```python
from build123d import *

# Parameters (mm, degrees)
SKETCH1_W           = 279.4
SKETCH1_H           = 376.174
BOSS_EXTRUDE1_DEPTH = 2.54
SKETCH2_W           = 28.448
SKETCH2_H           = 19.05
CUT_EXTRUDE1_DEPTH  = 235.305913645


with BuildPart() as part:
    # Sketch1 → Boss-Extrude1 (new body)
    with BuildSketch(Plane(origin=(0, 0, 0), x_dir=(1, 0, 0), z_dir=(0, 1, 0))):
        Rectangle(SKETCH1_W, SKETCH1_H)
    extrude(amount=BOSS_EXTRUDE1_DEPTH)

    # Sketch2 → Cut-Extrude1 (cut, through all)
    with BuildSketch(Plane(origin=(0, 2.54, 0), x_dir=(1, 0, 0), z_dir=(0, 1, 0))):
        with Locations((-120.65, -105.537)):
            Rectangle(SKETCH2_W, SKETCH2_H)
        with Locations((-120.65, -162.687)):
            Rectangle(SKETCH2_W, SKETCH2_H)
        with Locations((-120.65, -48.387)):
            Rectangle(SKETCH2_W, SKETCH2_H)
        with Locations((-120.65, 8.763)):
            Rectangle(SKETCH2_W, SKETCH2_H)
        with Locations((-120.65, 65.913)):
            Rectangle(SKETCH2_W, SKETCH2_H)
        with Locations((120.65, 65.913)):
            Rectangle(SKETCH2_W, SKETCH2_H)
        with Locations((120.65, 8.763)):
            Rectangle(SKETCH2_W, SKETCH2_H)
        with Locations((120.65, -48.387)):
            Rectangle(SKETCH2_W, SKETCH2_H)
        with Locations((120.65, -105.537)):
            Rectangle(SKETCH2_W, SKETCH2_H)
        with Locations((120.65, -162.687)):
            Rectangle(SKETCH2_W, SKETCH2_H)
    extrude(amount=-CUT_EXTRUDE1_DEPTH, mode=Mode.SUBTRACT)


solid = part.part
```
Part model, mm, in its own coordinate system. Round coordinates to 2 decimals unless told otherwise and drop trailing zeros. Loops run counter-clockwise (first coordinate to the right, second up) from the corner with the lowest first, then second, coordinate; pieces in that order, holes last.
Item 1: Cut at A-A, the plane z = -61.5. Give the cut face in (x, y), then the cut area to 3 significant figures.
Item 2: Cut at B-B, the plane y = 0.8. State how many separate pieces and enclosed holes the cut face has, then the cut area to 3 significant figures.
Item 3: Drill centre lines: line 1 (Z direction, x = 116, y = 1.45); line 2 (X direction, y = 1.8, z = 155). Where is each one in solid material? Low to high.
A:
1. outline: (-139.7, 0) - (-134.87, 0) - (-134.87, 2.54) - (-139.7, 2.54) - close; (-106.43, 0) - (106.43, 0) - (106.43, 2.54) - (-106.43, 2.54) - close; (134.87, 0) - (139.7, 0) - (139.7, 2.54) - (134.87, 2.54) - close
1. area: 565 mm2
2. separate pieces: 1
2. enclosed holes: 10
2. area: 99,700 mm2
3. line 1: z = -188.09 to -75.44, -56.39 to -18.29, 0.76 to 38.86, 57.91 to 96.01, 115.06 to 153.16, 172.21 to 188.09
3. line 2: x = -139.7 to -134.87, -106.43 to 106.43, 134.87 to 139.7
